Here's how the part is built. I have some questions about the finished solid (model axes, mm). A direction names the side the tool comes from. Coordinates: 2 decimals unless noted, no trailing zeros. Loops run counter-clockwise (first coordinate to the right, second up) from the corner with the lowest first, then second, coordinate; pieces in that order, holes last. Notation, with made-up numbers: (24.5, 72.5) -> (60.5, 72.5) arc R25 ccw to (60.5, 106.5) -> close; hole circle Ø11 at (-2, 82.5). An arc over 180 degrees is marked (long way). Answer as a JSON object with one key per item and string values. Group by question number.
1) I'm going to push flat-ended pins straight in: pin 1 (2.5 mm diameter, centred on x = 47.5, z = -48, fed in from +Y); pin 2 (0.6 mm diameter, centred on x = -49, z = -38.5, fed in from +Y). Where does each tip first touch, or does it pass through?
2) Which directions (+Z, -Z, +X, -X, +Y, -Y) give clear straight access to the entire face, cutting with the end or side of a thin tool? Please do faces 5 (the flat face through (48.3, 245, -48.3)), 6 (the flat face through (1, 123, 50)), 7 (the flat face through (48, 123, -1)).
3) If we mould it in two halves opening along Z, with no side actions, what happens to faces 1 (the flat face through (-1, 123, -50)), 2 (the flat face through (-48.2, 245, 48.3)), 3 (the flat face through (-1, 123, -48)), 4 (the flat face through (-50, 123, 1))? For each: +Z half, -Z half, draft (parallel to the pull), parting line (faces both ways), or undercut.
4) I want a section at C-C (x = -26). Write out the boundary of the cut face in (y, z), then the cut area to 3 significant figures.
5) I want a section at A-A (z = 32.5). Write out the boundary of the cut face in (x, y).
6) I need wall thicknesses on probe 1 along Z at (x, y) = (7, 69.5). Which ranges of the line are inside material? Lowest first, please. Write a range as [from, to].
7) I want a section at B-B (y = 58). Write out the boundary of the cut face in (x, z), then the cut area to 3 significant figures.
Autodesk Inventor part; units mm, degrees
ref_plane "Work Plane1" through (50, 104, 50) normal (-0.7071, 0, 0.7071) x (0, -1, 0)
ref_plane "Work Plane2" through (-48, 104, 50) normal (0.7071, 0, 0.7071) x (0, 1, 0)
ref_plane "YZ Plane" through (0, 0, 0) normal (1, 0, 0) x (0, 1, 0)
sketch "Sketch1" plane through (0, 0, 0) normal (0, 1, 0) x (-1, 0, 0)
  line L0 (-50, 50) -> (50, 50)
  line L1 (50, 50) -> (50, -50)
  line L2 (50, -50) -> (-50, -50)
  line L3 (-50, -50) -> (-50, 50)
  line L4 (-50, 50) -> (50, -50) construction
  line L5 (50, 50) -> (-50, -50) construction
  line L6 (-48, 48) -> (48, 48)
  line L7 (48, 48) -> (48, -48)
  line L8 (48, -48) -> (-48, -48)
  line L9 (-48, -48) -> (-48, 48)
  line L10 (-48, 48) -> (48, -48) construction
  line L11 (48, 48) -> (-48, -48) construction
  point P0 (0, 0)
  dimension "d0" = 100
  dimension "d1" = 100
  dimension "d2" = 2
extrude "Extrusion1" add sketch "Sketch1" along normal blind 250
sketch "Sketch3" plane through (50, 250, 50) normal (1, 0, 0) x (0, 0, -1)
  line L0 (2, 0) -> (98, 0)
  line L1 (10, 0) -> (12, 0)
  line L2 (12, 0) -> (12, -100)
  line L3 (12, -100) -> (10, -100)
  line L4 (10, -100) -> (10, 0)
  line L5 (0, -250) -> (0, 0)
  point P0 (50, -250)
  point P1 (0, -146)
  point P2 (12, 0)
  dimension "d9" = 100
  dimension "d10" = 2
  dimension "d11" = 10
extrude "Extrusion3" cut sketch "Sketch3" against normal blind 220
mirror "Mirror2" about plane through (0, 0, 0) normal (0, 0, 1) of "Extrusion3"
sketch "Sketch4" plane through (-50, 250, 50) normal (0, 0, 1) x (1, 0, 0)
  line L0 (10, 0) -> (12, 0)
  line L1 (12, 0) -> (12, -100)
  line L2 (12, -100) -> (10, -100)
  line L3 (10, -100) -> (10, 0)
  line L4 (0, -250) -> (0, 0)
  line L5 (0, 0) -> (100, 0)
  point P0 (50, -250)
  point P1 (0, -146)
  point P2 (10, -50)
  point P3 (11, 0)
  dimension "d14" = 10
  dimension "d15" = 2
  dimension "d16" = 100
  dimension "d17" = 0
extrude "Extrusion4" cut sketch "Sketch4" against normal blind 220
mirror "Mirror3" about plane through (0, 0, 0) normal (1, 0, 0) of "Extrusion4"
ref_plane "Work Plane1" through (50, 104, 50) normal (-0.7071, 0, 0.7071) x (0, -1, 0)
sketch "Sketch5" plane through (50, 104, 50) normal (-0.7071, 0, 0.7071) x (0, -1, 0)
  line L0 (-141, -72.7107) -> (-146, -72.7107)
  line L1 (-146, -72.7107) -> (-146, -68.7107)
  line L2 (-146, -68.7107) -> (-141, -68.7107)
  line L3 (-141, -68.7107) -> (-141, -72.7107)
  line L4 (-141, -72.7107) -> (-146, -68.7107) construction
  line L5 (-146, -72.7107) -> (-141, -68.7107) construction
  line L6 (104, -70.7107) -> (-146, -70.7107)
  point P0 (-143.5, -70.7107)
  point P1 (0, -70.7107)
  dimension "d20" = 5
  dimension "d21" = 4
  dimension "d22" = 0
  dimension "d23" = 0
extrude "Extrusion5" cut sketch "Sketch5" along normal mid plane 220
ref_plane "Work Plane2" through (-48, 104, 50) normal (0.7071, 0, 0.7071) x (0, 1, 0)
sketch "Sketch6" plane through (-48, 104, 50) normal (0.7071, 0, 0.7071) x (0, 1, 0)
  line L0 (141, -67.2965) -> (146, -67.2965)
  line L1 (146, -67.2965) -> (146, -71.2965)
  line L2 (146, -71.2965) -> (141, -71.2965)
  line L3 (141, -71.2965) -> (141, -67.2965)
  line L4 (-104, -69.2965) -> (146, -69.2965)
  line L5 (141, -67.2965) -> (146, -71.2965) construction
  line L6 (146, -67.2965) -> (141, -71.2965) construction
  line L7 (146, -62.2254) -> (146, -69.2965)
  point P0 (143.5, -69.2965)
  point P1 (0, -69.2965)
  dimension "d26" = 4
  dimension "d27" = 5
  dimension "d28" = 0
extrude "Extrusion6" cut sketch "Sketch6" along normal mid plane 220
properties part number "FLueExtension"
Determined:
{
 "1": {"pin 1": "y = 245", "pin 2": "y = 150"},
 "2": {"face 5": "+Y", "face 6": "+Z, +X, -X, +Y, -Y", "face 7": "+Y, -Y"},
 "3": {"face 1": "-Z half", "face 2": "undercut", "face 3": "undercut", "face 4": "draft"},
 "4": {"outline": "(0, -50) -> (250, -50) -> (250, -48) -> (0, -48) -> close; (0, 48) -> (250, 48) -> (250, 50) -> (0, 50) -> close", "area": "1,000 mm^2"},
 "5": {"outline": "(-50, 0) -> (-48, 0) -> (-48, 250) -> (-50, 250) -> close; (48, 0) -> (50, 0) -> (50, 250) -> (48, 250) -> close"},
 "6": {"probe 1": "[-50, -48], [48, 50]"},
 "7": {"outline": "(-50, -50) -> (50, -50) -> (50, 50) -> (-50, 50) -> close; hole (-48, -48) -> (48, -48) -> (48, 48) -> (-48, 48) -> close", "area": "784 mm^2"}
}
